Autodesk Inventor part; units mm, degrees
ref_plane "РабПлоскость1" through (20, 3, 15) normal (0, -1, 0) x (1, 0, 0)
ref_plane "РабПлоскость2" through (-20, 17, 0) normal (0, -1, 0) x (1, 0, 0)
ref_plane "YZ Plane" through (0, 0, 0) normal (1, 0, 0) x (0, 1, 0)
sketch "Эскиз1" plane through (0, 0, 0) normal (0, 0, 1) x (1, 0, 0)
  line L0 (-20, 0) -> (20, 0)
  line L1 (20, 0) -> (20, 3)
  line L2 (20, 3) -> (5.5172, 16.7931)
  line L3 (0, 0) -> (0, 19)
  line L4 (-20, 0) -> (-20, 3)
  line L5 (-20, 3) -> (-5.5172, 16.7931)
  arc A0 (5.5172, 16.7931) -> (-5.5172, 16.7931) centre (0, 11) ccw
  dimension "d0" = 40
  dimension "d1" = 3
  dimension "d2" = 8
  dimension "d3" = 11
extrude "Выдавливание1" add sketch "Эскиз1" along normal blind 15
ref_plane "РабПлоскость1" through (20, 3, 15) normal (0, -1, 0) x (1, 0, 0)
sketch "Эскиз2" plane through (20, 3, 15) normal (0, -1, 0) x (1, 0, 0)
  line L0 (-40, -15) -> (-40, 0)
  line L1 (-40, -13) -> (-30, -13)
  line L2 (-30, -13) -> (-30, -2)
  line L3 (-30, -2) -> (-40, -2)
  line L4 (-40, -2) -> (-40, -13)
  line L5 (0, -15) -> (0, 0)
  line L6 (0, -13) -> (-10, -13)
  line L7 (-10, -13) -> (-10, -2)
  line L8 (-10, -2) -> (0, -2)
  line L9 (0, -2) -> (0, -13)
  line L10 (-40, -7.5) -> (0, -7.5)
  line L11 (-20, -15) -> (-20, 0)
  line L12 (-40, 0) -> (0, 0)
  point P0 (-10, -7.5)
  point P1 (-30, -7.5)
  point P2 (-40, -7.5)
  dimension "d6" = 20
  dimension "d7" = 11
extrude "Выдавливание2" cut sketch "Эскиз2" against normal through all contours L0 L10 L2 L1 | L0 L3 L2 L10 | L10 L5 L6 L7 | L7 L8 L5 L10
sketch "Эскиз3" plane through (20, 3, 15) normal (0, 1, 0) x (1, 0, 0)
  line L0 (-40, 13) -> (-40, 2)
  line L1 (-20, 15) -> (-20, 0)
  line L2 (-40, 0) -> (0, 0)
  point P0 (-35, 7.5)
  point P1 (-5, 7.5)
  point P2 (-40, 7.5)
  dimension "d17" = 30
hole "Отверстие1" at (-15, 3, 7.5) at (15, 3, 7.5) direction (0, -1, 0) diameter 3.3 end through all countersink diameter 5 countersink angle 90
ref_plane "РабПлоскость2" through (-20, 17, 0) normal (0, -1, 0) x (1, 0, 0)
sketch "Эскиз5" plane through (-20, 17, 0) normal (0, -1, 0) x (1, 0, 0)
  line L0 (0, 2) -> (10, 2)
  line L1 (30, 13) -> (30, 2)
  line L2 (10, 2) -> (30, 2)
  line L3 (30, 2) -> (30, 13)
  line L4 (30, 13) -> (10, 13)
  line L5 (10, 13) -> (10, 2)
  point P0 (20, 0)
extrude "Выдавливание3" cut sketch "Эскиз5" against normal through all
sketch "Эскиз6" plane through (0, 0, 15) normal (0, 0, 1) x (1, 0, 0)
  arc A0 (5.5172, 16.7931) -> (-5.5172, 16.7931) centre (0, 11) ccw
  arc A1 (-1.9621, 12.2) -> (1.9621, 12.2) centre (0, 11) ccw
  line L0 (-1.9621, 12.2) -> (1.9621, 12.2)
  point P0 (0, 0)
  dimension "d32" = 2.3
  dimension "d33" = 1.2
extrude "Выдавливание4" cut sketch "Эскиз6" against normal through all
sketch "Эскиз7" plane through (-20, 17, 0) normal (0, 1, 0) x (1, 0, 0)
  line L0 (14.7085, -13) -> (14.7085, -2)
  line L1 (14.7085, -13) -> (25.2915, -13)
  point P0 (20, 0)
  point P1 (20, -7.5)
  point P2 (14.7085, -7.5)
  point P3 (20, -13)
hole "Отверстие3" at (0, 17, 7.5) direction (0, -1, 0) diameter 2.8 depth 4.8
properties part number "engine_center"
For this review, take the finished solid that the model builds, in its own axes (mm). A direction names the side the tool comes from. Round coordinates to 2 decimals unless told otherwise and drop trailing zeros. Order: outer loops, then holes, each group sorted by start corner. A loop starts at its lowest first (then second) coordinate and runs counter-clockwise, first axis right, second up. Notation, with made-up numbers: (2, -36.75) -> (24, -36.75) arc R20 cw to (24, -24.75) -> close; hole circle Ø3 at (40, 20.25). An arc over 180 degrees is marked (long way). Use a Markdown table: item, result.
Item 1: Take a section at C-C (y = 9.5). State the section outline as (x, z) points, plus the area to 3 significant figures.
Resolved:
| item | result |
|---|---|
| outline | (-13.17, 0) -> (-1.74, 0) -> (-1.74, 15) -> (-13.17, 15) -> (-13.17, 13) -> (-10, 13) -> (-10, 2) -> (-13.17, 2) -> close; (1.74, 0) -> (13.17, 0) -> (13.17, 2) -> (10, 2) -> (10, 13) -> (13.17, 13) -> (13.17, 15) -> (1.74, 15) -> close |
| area | 273 mm² |
Item 2: Draft analysis for pull direction Z (two halves, no side actions). For faces 1 (the flat face through (10, 8, 7)), 2 (the flat face through (0, 8, 0)), 3 (the cylindrical face through (-0.07, 8.7, 7.6)), state which applies: +Z half, -Z half, draft (parallel to the pull), parting line (faces both ways), or undercut.
Resolved:
| item | result |
|---|---|
| face 1 | undercut |
| face 2 | -Z half |
| face 3 | draft |
Item 3: Take a section at D-D (z = 7.5). State how many separate pieces and enclosed holes the cut face has, plus the area to 3 significant figures.
Resolved:
| item | result |
|---|---|
| separate pieces | 3 |
| enclosed holes | 0 |
| area | 331 mm² |
Item 4: Take a section at B-B (x = 0). State the section outline as (y, z) points.
Resolved:
| item | result |
|---|---|
| outline | (0, 0) -> (8.7, 0) -> (8.7, 15) -> (0, 15) -> close; (12.2, 0) -> (19, 0) -> (19, 2) -> (17, 2) -> (17, 6.1) -> (12.2, 6.1) -> close; (12.2, 8.9) -> (17, 8.9) -> (17, 13) -> (19, 13) -> (19, 15) -> (12.2, 15) -> close |
Item 5: For line 1 along X through (y, z) = (0.9, 7.5); line 2 along Z through (x, y) = (15, 0.9); line 3 along Y through (x, z) = (0, 4.75), list the stretches that pass through material, from the lowest coordinate up. Write a range as [from, to].
Resolved:
| item | result |
|---|---|
| line 1 | x = [-20, -16.65], [-13.35, 13.35], [16.65, 20] |
| line 2 | z = [0, 5.85], [9.15, 15] |
| line 3 | y = [0, 8.7], [12.2, 17] |
Item 6: For pin 1 (2 mm diameter, centred on x = 15, z = 7.5, fed in from -Y); pin 2 (7.5 mm diameter, centred on y = 9, z = 6.5, fed in from -X); pin 3 (5.5 mm diameter, centred on x = -0.5, z = 8.5, fed in from +Y); pin 4 (3 mm diameter, centred on y = 8, z = 8, fed in from +X), all flat-tipped, find the tip position at first contact; note any pin that passes through.
Resolved:
| item | result |
|---|---|
| pin 1 | passes through |
| pin 2 | stops at x = -10 |
| pin 3 | stops at y = 17 |
| pin 4 | stops at x = 10 |
Item 7: Machinability: for faces 4 (the flat face through (-16, 3, 10)), 5 (the flat face through (0, 12.2, 5.9)), 6 (the flat face through (14, 3, 10)), which of the approach directions +Z, -Z, +X, -X, +Y, -Y give a long, thin tool a straight path to every point of the face, cutting with its end or side? Answer none if there is none.
Resolved:
| item | result |
|---|---|
| face 4 | -X, +Y |
| face 5 | +Z, -Z |
| face 6 | +X, +Y |
Item 8: Take a section at A-A (z = 3.25). State the section outline as (x, y) points.
Resolved:
| item | result |
|---|---|
| outline | (-20, 0) -> (20, 0) -> (20, 3) -> (10, 3) -> (10, 12.52) -> (5.52, 16.79) arc R8 ccw to (5.29, 17) -> (-5.29, 17) arc R8 ccw to (-5.52, 16.79) -> (-10, 12.52) -> (-10, 3) -> (-20, 3) -> close; hole (-1.96, 12.2) arc R2.3 ccw (long way) to (1.96, 12.2) -> close |
